from build123d import *

# Parameters (mm, degrees)
F1_DEPTH       = 15
F2_R           = 2
F3_DEPTH       = 25
F5_D           = 4
F5_CSINK_D     = 7
F5_CSINK_ANGLE = 90


with BuildPart() as f1:
    # F0 (on Top) → F1 (new body)
    with BuildSketch(Plane.XY):
        Polygon((0, 3), (0, 0), (15, 0), (15, 9), (41, 9), (41, 0), (56, 0), (56, 3), (44, 3), (44, 12), (12, 12), (12, 3), align=None)
    extrude(amount=F1_DEPTH)

    # F2 (on face) → F3 (cut)
    with BuildSketch(Plane(origin=(0, 12, 0), x_dir=(-1, 0, 0), z_dir=(0, 1, 0))):
        with Locations((-36, 11)):
            Circle(F2_R)
        with Locations((-20, 11)):
            Circle(F2_R)
    extrude(amount=-F3_DEPTH, mode=Mode.SUBTRACT)

    # F5 (through all)
    with Locations(Plane(origin=(0, 3, 0), x_dir=(-1, 0, 0), z_dir=(0, 1, 0))):
        with Locations((-6, 5), (-50, 5)):
            CounterSinkHole(F5_D / 2, F5_CSINK_D / 2, counter_sink_angle=F5_CSINK_ANGLE)


solid = f1.part
Design review of the part built by this model. Coordinates are the model's own, in mm. A direction names the side the tool comes from. Give positions to 0.01 mm unless a question says otherwise; leave off trailing zeros. Write each loop counter-clockwise with the first axis right and the second up, starting at its lowest first coordinate (ties: lowest second). Pieces come first, ordered by that corner, then holes. Notation, with made-up numbers: M 59,15 L 83,15 A26 ccw 83,47 Z; hole C 59,87 d9. An arc over 180 degrees is marked long. Return JSON: item names as keys, results as strings. Group by question number.
Item 1: Wall thickness on line 1 along X through (y, z) = (0.5, 5); line 2 along Z through (x, y) = (6, 0.9); line 3 along X through (y, z) = (6, 4): over which ranges is each line inside the solid? List them lowest first.
Item 2: Take a section at A-A (x = 6). Give the boundary of the cut face in (y, z), plus the area to 4 significant figures.
Item 3: Tool access review of faces 1 (the flat face through (28, 9, 7)), 2 (the flat face through (28, 12, 7)), 3 (the flat face through (12, 8, 7)), 4 (the flat face through (50, 3, 9)), 5 (the flat face through (48, 0, 7)): name each direction out of +Z, -Z, +X, -X, +Y, -Y from which nothing blocks a thin tool from reaching the whole face with its end or side.
Item 4: Clearance check with flat-ended pins moving along their axes: pin 1 Ø5 at (y, z) = (8, 2) entering from +X; pin 2 Ø2.5 at (y, z) = (6, 8) entering from -X; pin 3 Ø5 at (x, z) = (36, 11) entering from -Y. State where each tip first meets the part, or that it passes through.
Item 5: Take a section at D-D (x = 36). Give the boundary of the cut face in (y, z).
Item 6: Take a section at B-B (y = 5). Give the boundary of the cut face in (x, z).
Item 7: The part is to be moulded in two halves that separate along Z. For faces 6 (the cylindrical face through (36, 11, 13)), 7 (the flat face through (28, 10, 15)), 8 (the flat face through (41, 5, 7)), say which applies: pulls with the +Z half, pulls with the -Z half, needs draft (parallel to the pull), parting line crosses it, or undercut.
Item 8: Take a section at C-C (z = 11). Give the boundary of the cut face in (x, y).
Return value:
{
 "1": {"line 1": "x = 0 to 4, 8 to 15, 41 to 48, 52 to 56", "line 2": "z = 0 to 3, 7 to 15", "line 3": "x = 12 to 15, 41 to 44"},
 "2": {"outline": "M 0,0 L 3,0 L 3,1.5 L 1.5,3 L 0,3 Z; M 0,7 L 1.5,7 L 3,8.5 L 3,15 L 0,15 Z", "area": "30.75 mm2"},
 "3": {"face 1": "+Z, -Z, -Y", "face 2": "+Z, -Z, +X, -X, +Y", "face 3": "+Z, -Z, -X, +Y", "face 4": "+Z, -Z, +X, +Y", "face 5": "+Z, -Z, +X, -X, -Y"},
 "4": {"pin 1": "stops at x = 44", "pin 2": "stops at x = 12", "pin 3": "stops at y = 9"},
 "5": {"outline": "M 9,0 L 12,0 L 12,9 L 9,9 Z; M 9,13 L 12,13 L 12,15 L 9,15 Z"},
 "6": {"outline": "M 12,0 L 15,0 L 15,15 L 12,15 Z; M 41,0 L 44,0 L 44,15 L 41,15 Z"},
 "7": {"face 6": "undercut", "face 7": "pulls with the +Z half", "face 8": "needs draft"},
 "8": {"outline": "M 0,0 L 15,0 L 15,9 L 18,9 L 18,12 L 12,12 L 12,3 L 0,3 Z; M 22,9 L 34,9 L 34,12 L 22,12 Z; M 38,9 L 41,9 L 41,0 L 56,0 L 56,3 L 44,3 L 44,12 L 38,12 Z"}
}
